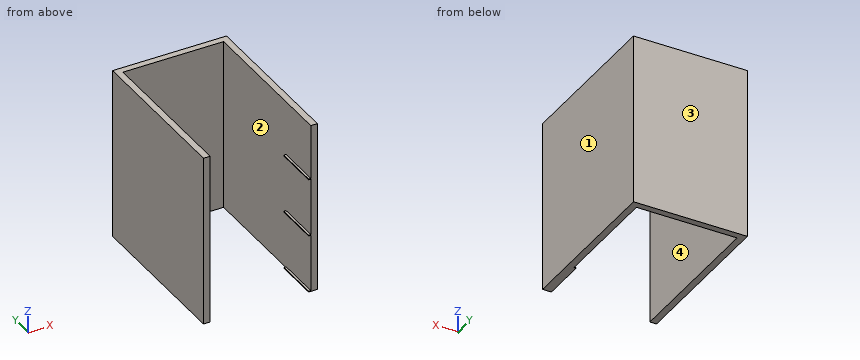
```python
from build123d import *

# Parameters (mm, degrees)
F1_DEPTH = 495.3
F2_W     = 6.35
F2_H     = 2.54
F3_DEPTH = 127


with BuildPart() as f1:
    # F0 (on Top) → F1 (new body)
    with BuildSketch(Plane.XY):
        Polygon((-257.175, 12.7), (12.7, 12.7), (22.86, 12.7), (22.86, -434.975), (41.91, -434.975), (41.91, 31.75), (-286.385, 31.75), (-286.385, -434.975), (-267.335, -434.975), (-267.335, 12.7), align=None)
    extrude(amount=F1_DEPTH)

    # F2 (on face) → F3 (join)
    with BuildSketch(Plane.XZ.offset(434.975)):
        with Locations((19.685, 1.27)):
            Rectangle(F2_W, F2_H)
        with Locations((19.685, 168.91)):
            Rectangle(F2_W, F2_H)
        with Locations((19.685, 336.55)):
            Rectangle(F2_W, F2_H)
    extrude(amount=-F3_DEPTH)


solid = f1.part
```
Source: CAD feature listing. Evaluate the final solid. Frame: model axes, mm. Face numbers are marked on the shaded views. A direction names the side the tool comes from. Round coordinates to 2 decimals unless told otherwise and drop trailing zeros. Loops run counter-clockwise (first coordinate to the right, second up) from the corner with the lowest first, then second, coordinate; pieces in that order, holes last.
1. Section query D-D on x = -37.5. Output: boundary loops of the cut face in (y, z).
2. Section query C-C on y = -67. Output: boundary loops of the cut face in (x, z) (3 decimals), and give its area (3 significant figures).
3. Contact query for flat-ended pins moving along their axis: pin 1 (1.9 mm diameter, centred on x = 21, y = -348, fed in from -Z); pin 2 (4 mm diameter, centred on x = -72, z = 310.5, fed in from -Y). Output: stop coordinate, or through.
4. Section query B-B on z = 84. Output: boundary loops of the cut face in (x, y) (3 decimals), and give its area (3 significant figures).
5. Access query for the marked faces 3 and 4. Directions: +Z, -Z, +X, -X, +Y, -Y. A direction counts if a zero-diameter tool reaches every point of the face in a straight line with its end or side. Return the directions, or none.
6. Ray query, L1, parallel to X at y = -66, z = 191 (3 decimals); L2, parallel to Y at x = -49, z = 105. Return the intervals inside material, ascending.
7. Mould query, pull axis Z, two halves, no side actions, for the marked faces 1 and 2. Classes: released by +Z, released by -Z, zero draft, split by the parting line, or undercut.
8. Section query A-A on y = -390.5. Output: boundary loops of the cut face in (x, z) (3 decimals), and give its area (3 significant figures).
Answers below:
1. outline: (12.7, 0) - (31.75, 0) - (31.75, 495.3) - (12.7, 495.3) - close
2. outline: (-286.385, 0) - (-267.335, 0) - (-267.335, 495.3) - (-286.385, 495.3) - close; (22.86, 0) - (41.91, 0) - (41.91, 495.3) - (22.86, 495.3) - close
2. area: 18,900 mm2
3. pin 1: stops at z = 0
3. pin 2: stops at y = 12.7
4. outline: (-286.385, -434.975) - (-267.335, -434.975) - (-267.335, 12.7) - (22.86, 12.7) - (22.86, -434.975) - (41.91, -434.975) - (41.91, 31.75) - (-286.385, 31.75) - close
4. area: 23,300 mm2
5. face 3: +Z, -Z, +X, -X, +Y
5. face 4: +Z, -Z, -Y
6. L1: x = -286.385 to -267.335, 22.86 to 41.91
6. L2: y = 12.7 to 31.75
7. face 1: zero draft
7. face 2: undercut
8. outline: (-286.385, 0) - (-267.335, 0) - (-267.335, 495.3) - (-286.385, 495.3) - close; (16.51, 0) - (41.91, 0) - (41.91, 495.3) - (22.86, 495.3) - (22.86, 337.82) - (16.51, 337.82) - (16.51, 335.28) - (22.86, 335.28) - (22.86, 170.18) - (16.51, 170.18) - (16.51, 167.64) - (22.86, 167.64) - (22.86, 2.54) - (16.51, 2.54) - close
8. area: 18,900 mm2
